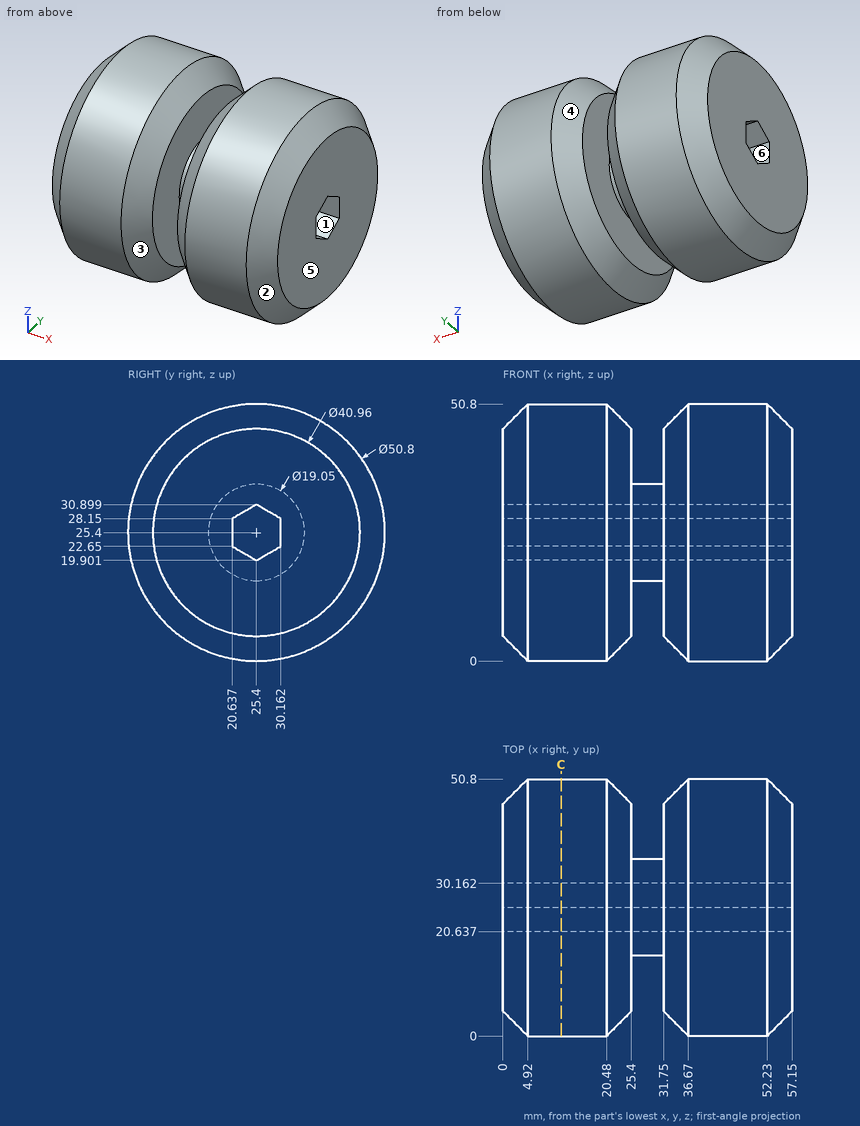
Input: dimensioned drawing with shaded views. Units: mm. Origin: part minimum x, y, z. A direction names the side the tool comes from. Round coordinates to 2 decimals unless told otherwise and drop trailing zeros. Loops run counter-clockwise (first coordinate to the right, second up) from the corner with the lowest first, then second, coordinate; pieces in that order, holes last.
1) Pull-direction query (X, two-part tool) for the marked faces 4, 5 and 6; classes: released by +X, released by -X, zero draft, split by the parting line, or undercut.
Ans:
face 4: undercut
face 5: released by +X
face 6: zero draft
2) Section query C-C on x = 11.5. Return the cut outline in (y, z), plus the area to 3 significant figures.
Ans:
outline: circle Ø50.8 at (25.4, 25.4); hole (20.64, 22.65) - (25.4, 19.9) - (30.16, 22.65) - (30.16, 28.15) - (25.4, 30.9) - (20.64, 28.15) - close
area: 1,950 mm2
3) Material intervals for line 1 (X direction, y = 16.5, z = 34); line 2 (Z direction, x = 48.5, y = 28) (1 decimal); line 3 (Z direction, x = 22.5, y = 28) (1 decimal), sorted ascending.
Ans:
line 1: x = 0 to 25.4, 31.75 to 57.15
line 2: z = 0.1 to 21.4, 29.4 to 50.7
line 3: z = 2.2 to 21.4, 29.4 to 48.6
4) Set-up query: the marked faces 1, 2 and 3. Return all of +Z, -Z, +X, -X, +Y, -Y with unobstructed straight access to the full face (end or side cutting, diameter ignored); none if empty.
Ans:
face 1: +X, -X
face 2: +X
face 3: none
5) Pin query (flat end, axial travel): pin 1 (1 mm diameter, centred on y = 6, z = 14, fed in from -X); pin 2 (3 mm diameter, centred on x = 32.5, y = 6.5, fed in from +Z) (1 decimal); pin 3 (10 mm diameter, centred on x = 43.5, z = 22.5, fed in from +Y); pin 4 (20.5 mm diameter, centred on y = 22.5, z = 25, fed in from +X). Return the tip coordinate at first contact, or that it passes through.
Ans:
pin 1: stops at x = 1.52
pin 2: stops at z = 38.8
pin 3: stops at y = 50.8
pin 4: stops at x = 57.15
